```python
from build123d import *

# Parameters (mm, degrees)
BOSS_EXTRUDE1_DEPTH      = 7.5
BOSS_EXTRUDE1_DEPTH_BACK = 7.5
SKETCH1_R                = 30
SKETCH1_R_2              = 10.5
SKETCH1_R_3              = 2.5
CUT_EXTRUDE2_START       = 20
SKETCH2_R                = 2.1
CUT_EXTRUDE2_DEPTH       = 10


with BuildPart() as part:
    # Sketch1 → Boss-Extrude1 (new, two sides: drawn at the far end of the back side and taken through both)
    with BuildSketch(Plane(origin=(0, 0, 0), x_dir=(1, 0, 0), z_dir=(0, 1, 0)).offset(-BOSS_EXTRUDE1_DEPTH_BACK)):
        with Locations(Location((0, 0, 0), (0, 0, 270))):
            Circle(SKETCH1_R)
        with Locations(Location((0, 0, 0), (0, 0, 270))):
            Circle(SKETCH1_R_2, mode=Mode.SUBTRACT)
        with Locations(Location((17.67766953, 17.67766953, 0), (0, 0, 270))):
            Circle(SKETCH1_R_3, mode=Mode.SUBTRACT)
        with Locations(Location((17.67766953, -17.67766953, 0), (0, 0, 270))):
            Circle(SKETCH1_R_3, mode=Mode.SUBTRACT)
        with Locations(Location((-17.67766953, -17.67766953, 0), (0, 0, 270))):
            Circle(SKETCH1_R_3, mode=Mode.SUBTRACT)
        with Locations(Location((-17.67766953, 17.67766953, 0), (0, 0, 270))):
            Circle(SKETCH1_R_3, mode=Mode.SUBTRACT)
    extrude(amount=BOSS_EXTRUDE1_DEPTH + BOSS_EXTRUDE1_DEPTH_BACK)

    # Sketch2 → Cut-Extrude2 (cut)
    with BuildSketch(Plane.XY.offset(CUT_EXTRUDE2_START)):
        with Locations(Location((0, 0, 0), (0, 0, 270))):
            Circle(SKETCH2_R)
    extrude(amount=CUT_EXTRUDE2_DEPTH, mode=Mode.SUBTRACT)


solid = part.part
```
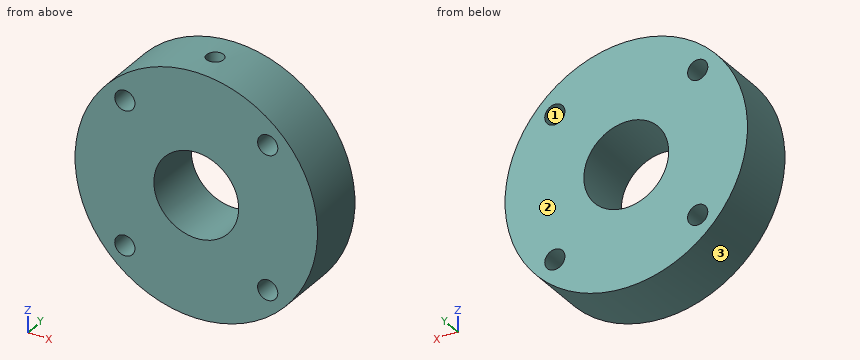
Source: CAD feature listing. Evaluate the final solid. Frame: model axes, mm. Face numbers are marked on the shaded views. Round coordinates to 2 decimals unless told otherwise and drop trailing zeros. Loops run counter-clockwise (first coordinate to the right, second up) from the corner with the lowest first, then second, coordinate; pieces in that order, holes last. Notation, with made-up numbers: M 70.25,55.25 L 74.25,55.25 A21 cw 74.25,70.25 Z; hole C 79.5,45.25 d10. An arc over 180 degrees is marked long. Put each result on its own line as item: value.
(1) First-contact query: pin 1 (4 mm diameter, centred on x = -17.68, z = 17.68, fed in from +Y); pin 2 (6 mm diameter, centred on y = -2, z = -5.5, fed in from -X); pin 3 (8 mm diameter, centred on x = 16.5, y = -5, fed in from +Z); pin 4 (1.3 mm diameter, centred on x = -0.5, y = -1, fed in from +Z). Flat tips, straight axial feed; report the tip coordinate or a pass-through.
Solutions:
pin 1: through
pin 2: x = -29.9
pin 3: z = 27.27
pin 4: z = 20
(2) Ray query, line 1 (X direction, y = 5, z = -17); line 2 (X direction, y = 5.5, z = -16); line 3 (Z direction, x = -9.5, y = 5.75). Return the intervals inside material, ascending. Write a range as [from, to].
Solutions:
line 1: [-24.72, -20.08], [-15.27, 15.27], [20.08, 24.72]
line 2: [-25.38, -19.53], [-15.82, 15.82], [19.53, 25.38]
line 3: [-28.46, -4.47], [4.47, 28.46]
(3) Section A-A, the plane x = 0. Return loops of the section in (y, z).
Solutions:
outline: M -7.5,-30 L 7.5,-30 L 7.5,-10.5 L -7.5,-10.5 Z; M -7.5,10.5 L 7.5,10.5 L 7.5,30 L 2.1,30 L 2.1,20 L -2.1,20 L -2.1,30 L -7.5,30 Z
(4) Pull-direction query (X, two-part tool) for the marked faces 1, 2 and 3; classes: released by +X, released by -X, zero draft, split by the parting line, or undercut.
Solutions:
face 1: undercut
face 2: zero draft
face 3: split by the parting line
(5) Section D-D, the plane z = 24.5. Return loops of the section in (x, y).
Solutions:
outline: M -17.31,-7.5 L 17.31,-7.5 L 17.31,7.5 L -17.31,7.5 Z; hole C 0,0 d4.2
(6) Section C-C, the plane y = 0. Return loops of the section in (x, z).
Solutions:
outline: M -2.1,20 L -2.1,29.93 A30 ccw long 2.1,29.93 L 2.1,20 Z; hole C -17.68,-17.68 d5; hole C -17.68,17.68 d5; hole C 0,0 d21; hole C 17.68,-17.68 d5; hole C 17.68,17.68 d5
(7) Section B-B, the plane z = 0. Return loops of the section in (x, y).
Solutions:
outline: M -30,-7.5 L -10.5,-7.5 L -10.5,7.5 L -30,7.5 Z; M 10.5,-7.5 L 30,-7.5 L 30,7.5 L 10.5,7.5 Z
